Verification items for the finished model (mm, model axes). A direction names the side the tool comes from. Round coordinates to 2 decimals unless told otherwise and drop trailing zeros. Write each loop counter-clockwise with the first axis right and the second up, starting at its lowest first coordinate (ties: lowest second). Pieces come first, ordered by that corner, then holes.
from build123d import *

# Parameters (mm, degrees)
IZIM1_R                     = 150
IZIM1_R_2                   = 130
Y_KSEKLIK_EKSTR_ZYON1_DEPTH = 300
IZIM2_W                     = 75
IZIM2_H                     = 60
KES_EKSTR_ZYON1_DEPTH       = 180


with BuildPart() as part:
    # Çizim1 → Yükseklik-Ekstrüzyon1 (new body)
    with BuildSketch(Plane(origin=(0, 0, 0), x_dir=(1, 0, 0), z_dir=(0, 1, 0))):
        with Locations(Location((0, 0, 0), (0, 0, 270))):
            Circle(IZIM1_R)
        with Locations(Location((0, 0, 0), (0, 0, 270))):
            Circle(IZIM1_R_2, mode=Mode.SUBTRACT)
    extrude(amount=Y_KSEKLIK_EKSTR_ZYON1_DEPTH)

    # Çizim2 → Kes-Ekstrüzyon1 (cut)
    with BuildSketch(Plane.XY):
        with Locations((-37.5, 30)):
            Rectangle(IZIM2_W, IZIM2_H)
        with Locations((37.5, 30)):
            Rectangle(IZIM2_W, IZIM2_H)
    extrude(amount=KES_EKSTR_ZYON1_DEPTH, mode=Mode.SUBTRACT)


solid = part.part
Q1. Sectioned sample at C-C (y = 247). Enter the section's corners in (x, z), plus the area to 3 significant figures.
Recorded:
outline: circle Ø300 at (0, 0); hole circle Ø260 at (0, 0)
area: 17,600 mm2
Q2. Depth check by flat-ended pin: P1, Ø10, axis at y = 86, z = -64, coming from the +X side; P2, Ø7, axis at y = 40, z = 121.5, coming from the +X side; P3, Ø7, axis at y = 23.5, z = 123.5, coming from the -X side. Enter the tip coordinate at first touch or a pass-through.
Recorded:
P1: stops at x = 137.91
P2: stops at x = 92.61
P3: stops at x = -90
Q3. Release check for a two-part mould opening along Z. For faces 1 (the flat face through (75, 30, 118)), 2 (the cylindrical face through (5.716, 147.9, -129.874)), 3 (the cylindrical face through (6.595, 147.9, -149.855)) record: released by +Z, released by -Z, zero draft, split by the parting line, or undercut.
Recorded:
face 1: zero draft
face 2: undercut
face 3: split by the parting line
Q4. Sectioned sample at D-D (z = 111). Enter the section's corners in (x, y), plus the area to 3 significant figures.
Recorded:
outline: (-100.89, 0) - (-75, 0) - (-75, 60) - (-67.67, 60) - (-67.67, 300) - (-100.89, 300) - close; (67.67, 60) - (75, 60) - (75, 0) - (100.89, 0) - (100.89, 300) - (67.67, 300) - close
area: 19,100 mm2
Q5. Sectioned sample at B-B (x = 0). Enter the section's corners in (y, z), plus the area to 3 significant figures.
Recorded:
outline: (0, -150) - (300, -150) - (300, -130) - (0, -130) - close; (60, 130) - (300, 130) - (300, 150) - (60, 150) - close
area: 10,800 mm2
Q6. Sectioned sample at A-A (z = 0). Enter the section's corners in (x, y), plus the area to 3 significant figures.
Recorded:
outline: (-150, 0) - (-130, 0) - (-130, 300) - (-150, 300) - close; (130, 0) - (150, 0) - (150, 300) - (130, 300) - close
area: 12,000 mm2
Q7. Tool access check on faces 4 (the flat face through (1, 60, 133)), 5 (the flat face through (123, 300, -45)). Record the directions out of +Z, -Z, +X, -X, +Y, -Y that give a thin tool (end or side, any length) a straight path to the whole face; none if there is none.
Recorded:
face 4: +Z, -Y
face 5: +Z, -Z, +X, -X, +Y
Q8. Material ranges on line 1 along Z through (x, y) = (0, 72.5); line 2 along X through (y, z) = (144, 73), recorded low to high.
Recorded:
line 1: z = -150 to -130, 130 to 150
line 2: x = -131.04 to -107.57, 107.57 to 131.04
